```python
from build123d import *

# Parameters (mm, degrees)
F0_R     = 3.175
F0_W     = 5.842
F0_H     = 12.7
F1_DEPTH = 13.6652


with BuildPart() as f1:
    # F0 (on Front) → F1 (new body)
    with BuildSketch(Plane.XZ):
        Polygon((5.842, 12.7), (5.842, 0), (66.294, 0), (66.294, 12.7), (56.134, 12.7), (56.134, 10.16), (10.16, 10.16), (10.16, 12.7), align=None)
        with BuildLine():
            ThreePointArc((-8.1826630726, -5.5069827884), (-3.1957909266, -4.5493385486), (-0.9398, 0))
            ThreePointArc((-0.9398, 0), (-4.5919612295, 5.3297205562), (-10.8806298187, 3.8475430269))
            ThreePointArc((-10.8806298187, 3.8475430269), (-12.1459778134, -1.5837270034), (-8.1826630726, -5.5069827884))
        make_face()
        with Locations((-6.6548, 0)):
            Circle(F0_R, mode=Mode.SUBTRACT)
        with BuildLine():
            Line((-0.9398, 0), (0, 0))
            Line((0, 0), (0, 12.7))
            Line((0, 12.7), (5.842, 12.7))
            Line((5.842, 12.7), (5.842, 15.24))
            Line((5.842, 15.24), (-0.508, 15.24))
            Line((-0.508, 15.24), (-10.8806298187, 3.8475430269))
            ThreePointArc((-10.8806298187, 3.8475430269), (-4.5919612295, 5.3297205562), (-0.9398, 0))
        make_face()
        with Locations((2.921, 6.35)):
            Rectangle(F0_W, F0_H)
        with BuildLine():
            Line((5.842, 0), (0, 0))
            Line((0, 0), (-0.9398, 0))
            ThreePointArc((-0.9398, 0), (-3.1957909266, -4.5493385486), (-8.1826630726, -5.5069827884))
            Line((-8.1826630726, -5.5069827884), (5.842, -9.398))
            Line((5.842, -9.398), (5.842, 0))
        make_face()
        with Locations((-6.6548, 0)):
            Circle(F0_R)
    extrude(amount=F1_DEPTH)


solid = f1.part
```
Here's how the part is built. I have some questions about the finished solid (model axes, mm). A direction names the side the tool comes from. Coordinates: 2 decimals unless noted, no trailing zeros. Order: outer loops, then holes, each group sorted by start corner. A loop starts at its lowest first (then second) coordinate and runs counter-clockwise, first axis right, second up.
Item 1: If we section it at D-D, the plane z = -2: List the corners of the cut face in (x, y) for me.
Response values:
outline: (-12.01, -13.67) - (5.84, -13.67) - (5.84, 0) - (-12.01, 0) - close
Item 2: If we section it at A-A, the plane y = -10.5: List the corners of the cut face in (x, z) for me (3 decimals).
Response values:
outline: (-10.881, 3.848) arc R5.715 ccw to (-8.183, -5.507) - (5.842, -9.398) - (5.842, 0) - (66.294, 0) - (66.294, 12.7) - (56.134, 12.7) - (56.134, 10.16) - (10.16, 10.16) - (10.16, 12.7) - (5.842, 12.7) - (5.842, 15.24) - (-0.508, 15.24) - close
Item 3: Thinking about a two-plate mould opening in X: for faces 1 (the face through (33, -7, 10.16)), 2 (the face through (-12.168, -6.737, -1.505)), 3 (the face through (26, -13.665, 3)), which applies, pulls with the +X half, pulls with the -X half, needs draft (parallel to the pull), parting line crosses it, or undercut?
Response values:
face 1: undercut
face 2: pulls with the -X half
face 3: needs draft
Item 4: Which directions (+Z, -Z, +X, -X, +Y, -Y) give clear straight access to the entire face, cutting with the end or side of a thin tool? Please do faces 4 (the face through (8, -7, 12.7)), 5 (the face through (-5.622, -6.737, 9.624)), 6 (the face through (56.134, -7, 11)), 7 (the face through (5.842, -7, -5)).
Response values:
face 4: +Z, +X, +Y, -Y
face 5: +Z, -X, +Y, -Y
face 6: +Z, +Y, -Y
face 7: -Z, +X, +Y, -Y
Item 5: I'm going to push flat-ended pins straight in: pin 1 Ø7 at (x, y) = (21.5, -5.5) entering from -Z; pin 2 Ø2 at (x, y) = (39, -6) entering from +Z; pin 3 Ø0.8 at (y, z) = (-7, 14) entering from +X. Where does each tip first touch, or does it pass through?
Response values:
pin 1: stops at z = 0
pin 2: stops at z = 10.16
pin 3: stops at x = 5.84
Item 6: I need wall thicknesses on probe 1 along Z at (x, y) = (8, -3.25); probe 2 along Z at (x, y) = (33, -3.75); probe 3 along X at (y, z) = (-3.75, 11). Which ranges of each line are inside material? Lowest first, please.
Response values:
probe 1: z = 0 to 12.7
probe 2: z = 0 to 10.16
probe 3: x = -4.37 to 10.16, 56.13 to 66.29
Item 7: If we section it at C-C, the plane x = 22.5: List the corners of the cut face in (y, z) for me, then the cut area to 3 significant figures.
Response values:
outline: (-13.67, 0) - (0, 0) - (0, 10.16) - (-13.67, 10.16) - close
area: 139 mm2
Item 8: If we section it at B-B, the plane z = 11: List the corners of the cut face in (x, y) for me.
Response values:
outline: (-4.37, -13.67) - (10.16, -13.67) - (10.16, 0) - (-4.37, 0) - close; (56.13, -13.67) - (66.29, -13.67) - (66.29, 0) - (56.13, 0) - close
